from build123d import *

# Parameters (mm, degrees)
SKETCH1_W               = 24
SKETCH1_H               = 21
PCB_DEPTH               = 1.6
MOUNT_HOLE_1_DEPTH      = 32.930549635
MOUNT_HOLE_1_DEPTH_BACK = 32.930549635
SKETCH2_R               = 1.25
MOUNT_HOLE_2_DEPTH      = 32.930549635
MOUNT_HOLE_2_DEPTH_BACK = 32.930549635
SKETCH3_R               = 1.25
MX1508_IC_START         = 1.6
SKETCH4_W               = 6
SKETCH4_H               = 5
MX1508_IC_DEPTH         = 1.2
PINS_IN_START           = 1.6
SKETCH5_W               = 18
SKETCH5_H               = 2.5
PINS_IN_DEPTH           = 6
PINS_OUT_START          = 1.6
SKETCH6_W               = 16
SKETCH6_H               = 2.5
PINS_OUT_DEPTH          = 6


with BuildPart() as part:
    # Sketch1 → PCB (new body)
    with BuildSketch(Plane(origin=(0, 0, 0), x_dir=(1, 0, 0), z_dir=(0, 1, 0))):
        with Locations((12, 10.5)):
            Rectangle(SKETCH1_W, SKETCH1_H)
    extrude(amount=PCB_DEPTH)

    # Sketch2 → Mount_hole_1 (cut, two sides: drawn at the far end of the back side and taken through both)
    with BuildSketch(Plane(origin=(0, 0, 0), x_dir=(1, 0, 0), z_dir=(0, 1, 0)).offset(-MOUNT_HOLE_1_DEPTH_BACK)):
        with Locations(Location((2, 19, 0), (0, 0, 270))):
            Circle(SKETCH2_R)
    extrude(amount=MOUNT_HOLE_1_DEPTH + MOUNT_HOLE_1_DEPTH_BACK, mode=Mode.SUBTRACT)

    # Sketch3 → Mount_hole_2 (cut, two sides: drawn at the far end of the back side and taken through both)
    with BuildSketch(Plane(origin=(0, 0, 0), x_dir=(1, 0, 0), z_dir=(0, 1, 0)).offset(-MOUNT_HOLE_2_DEPTH_BACK)):
        with Locations(Location((22, 19, 0), (0, 0, 270))):
            Circle(SKETCH3_R)
    extrude(amount=MOUNT_HOLE_2_DEPTH + MOUNT_HOLE_2_DEPTH_BACK, mode=Mode.SUBTRACT)

    # Sketch4 → MX1508_IC (add)
    with BuildSketch(Plane(origin=(0, 0, 0), x_dir=(1, 0, 0), z_dir=(0, 1, 0)).offset(MX1508_IC_START)):
        with Locations((12, 10.5)):
            Rectangle(SKETCH4_W, SKETCH4_H)
    extrude(amount=MX1508_IC_DEPTH)

    # Sketch5 → Pins_in (add)
    with BuildSketch(Plane(origin=(0, 0, 0), x_dir=(1, 0, 0), z_dir=(0, 1, 0)).offset(PINS_IN_START)):
        with Locations((11, 2.25)):
            Rectangle(SKETCH5_W, SKETCH5_H)
    extrude(amount=PINS_IN_DEPTH)

    # Sketch6 → Pins_out (add)
    with BuildSketch(Plane(origin=(0, 0, 0), x_dir=(1, 0, 0), z_dir=(0, 1, 0)).offset(PINS_OUT_START)):
        with Locations((12, 16.25)):
            Rectangle(SKETCH6_W, SKETCH6_H)
    extrude(amount=PINS_OUT_DEPTH)


solid = part.part
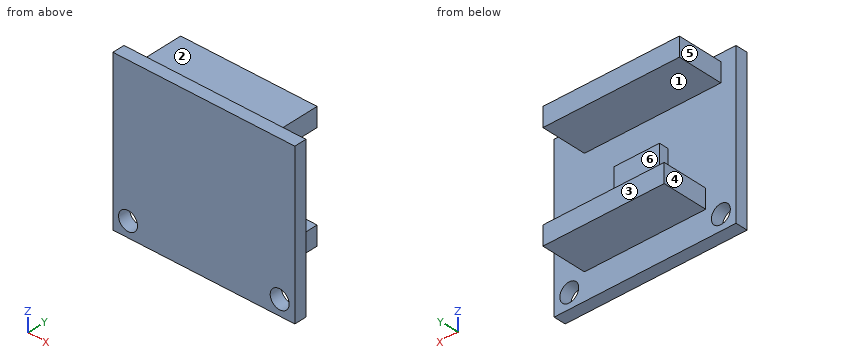
Geometry: final body of the model. Coordinates: model frame, mm. Face numbers are marked on the shaded views. A direction names the side the tool comes from. Round coordinates to 2 decimals unless told otherwise and drop trailing zeros. Order: outer loops, then holes, each group sorted by start corner. A loop starts at its lowest first (then second) coordinate and runs counter-clockwise, first axis right, second up. Notation, with made-up numbers: (-35.5, 57.25) -> (-29.5, 57.25) arc R14 ccw to (-29.5, 64.25) -> close; hole circle Ø6 at (7.25, 82.25). An arc over 180 degrees is marked (long way). Put each result on its own line as item: value. Start each with the question number.
Q1. Section C-C on x = 22. Return the cut outline in (y, z).
Q2. Line query: probe 1 along X at (y, z) = (0.45, -19); probe 2 along Z at (x, y) = (13, 6); probe 3 along Z at (x, y) = (2, 1.05). Output: solid intervals per line, ascending.
Q3. Pull-direction query (Z, two-part tool) for the marked faces 1, 2 and 3; classes: +Z half, -Z half, draft (parallel to the pull), parting line (faces both ways), or undercut.
Q4. Reachability of the marked faces 4, 5 and 6 from +Z, -Z, +X, -X, +Y, -Y: full face, straight path, thin tool, end or side. Return the list, or none.
Q5. First-contact query: pin 1 (1.2 mm diameter, centred on y = 5.5, z = -3, fed in from -X); pin 2 (4 mm diameter, centred on x = 22, z = -19, fed in from -Y); pin 3 (1.5 mm diameter, centred on x = 6, y = 4, fed in from -Z); pin 4 (3 mm diameter, centred on x = 9.5, y = 5.5, fed in from +Z). Flat tips, straight axial feed; report the tip coordinate or a pass-through.
Q6. Section A-A on y = 4.5. Return the cut outline in (x, z), and give its area (3 significant figures).
Q7. Section D-D on x = 7. Return the cut outline in (y, z), and give its area (3 significant figures).
Q8. Section B-B on z = -19. Return the cut outline in (x, y), and give its area (3 significant figures).
Ans:
1. outline: (0, -21) -> (1.6, -21) -> (1.6, -20.25) -> (0, -20.25) -> close; (0, -17.75) -> (1.6, -17.75) -> (1.6, 0) -> (0, 0) -> close
2. probe 1: x = 0 to 0.75, 3.25 to 20.75, 23.25 to 24
2. probe 2: z = -17.5 to -15, -3.5 to -1
2. probe 3: z = -21 to -20.25, -17.75 to 0
3. face 1: undercut
3. face 2: +Z half
3. face 3: draft
4. face 4: -Z, -X, +Y
4. face 5: +Z, -Z, -X, +Y
4. face 6: +X, -X, +Y
5. pin 1: stops at x = 2
5. pin 2: stops at y = 0
5. pin 3: stops at z = -17.5
5. pin 4: stops at z = -1
6. outline: (2, -3.5) -> (20, -3.5) -> (20, -1) -> (2, -1) -> close; (4, -17.5) -> (20, -17.5) -> (20, -15) -> (4, -15) -> close
6. area: 85.0 mm2
7. outline: (0, -21) -> (1.6, -21) -> (1.6, -17.5) -> (7.6, -17.5) -> (7.6, -15) -> (1.6, -15) -> (1.6, -3.5) -> (7.6, -3.5) -> (7.6, -1) -> (1.6, -1) -> (1.6, 0) -> (0, 0) -> close
7. area: 63.6 mm2
8. outline: (0, 0) -> (0.75, 0) -> (0.75, 1.6) -> (0, 1.6) -> close; (3.25, 0) -> (20.75, 0) -> (20.75, 1.6) -> (3.25, 1.6) -> close; (23.25, 0) -> (24, 0) -> (24, 1.6) -> (23.25, 1.6) -> close
8. area: 30.4 mm2
